Here's how the part is built. I have some questions about the finished solid (model axes, mm). A direction names the side the tool comes from. Round coordinates to 2 decimals unless told otherwise and drop trailing zeros. Order: outer loops, then holes, each group sorted by start corner. A loop starts at its lowest first (then second) coordinate and runs counter-clockwise, first axis right, second up. Notation, with made-up numbers: (-20.75, 15) -> (38.25, 15) arc R10 ccw to (38.25, 19) -> close; hole circle Ø9 at (68, 79). An arc over 180 degrees is marked (long way). Answer in a Markdown table with one row per item.
```python
from build123d import *

# Parameters (mm, degrees)
F0_W     = 80
F0_H     = 50
F1_DEPTH = 60
F2_SIZE  = 20
F4_D     = 16
F4_DEPTH = 10
F4_TIP   = 4.8068849522
F5_R     = 2
F6_R     = 2


with BuildPart() as f1:
    # F0 (on Top) → F1 (new body)
    with BuildSketch(Plane.XY):
        with Locations((40, 25)):
            Rectangle(F0_W, F0_H)
    extrude(amount=F1_DEPTH)

    # F2
    f2_edges = [f1.edges().sort_by_distance(p)[0] for p in [
        (40, 0, 60),
    ]]
    chamfer(f2_edges, length=F2_SIZE)

    # F4
    with Locations(Plane(origin=(0, -20, 20), x_dir=(1, 0, 0), z_dir=(0, -0.7071067812, 0.7071067812))):
        with Locations((20, 42.5685424949), (60, 42.5685424949)):
            Hole(F4_D / 2, depth=F4_DEPTH)
            with Locations((0, 0, -(F4_DEPTH + F4_TIP / 2))):  # 118° drill point
                Cone(0, F4_D / 2, F4_TIP, mode=Mode.SUBTRACT)

    # F5
    f5_edges = [f1.edges().sort_by_distance(p)[0] for p in [
        (80, 25, 0),
    ]]
    fillet(f5_edges, radius=F5_R)

    # F6
    f6_edges = [f1.edges().sort_by_distance(p)[0] for p in [
        (0, 25, 0),
    ]]
    fillet(f6_edges, radius=F6_R)


solid = f1.part
```
1. For faces 5 (the face through (20.75, 20.81, 41.05)), 6 (the face through (39, 10, 50)), which set-ups out of +Z, -Z, +X, -X, +Y, -Y let a thin tool reach every point of the face, with its end or its side?
Numbers:
| item | result |
|---|---|
| face 5 | none |
| face 6 | +Z, +X, -X, -Y |
2. Suppose I cut it at A-A on x = 72. Write out the boundary of the cut face in (y, z).
Numbers:
| item | result |
|---|---|
| outline | (0, 0) -> (50, 0) -> (50, 60) -> (20, 60) -> (0, 40) -> close |
3. We'd pull the mould along X, two halves only. Please class faces 1 (the face through (79.4, 25.35, 0.57)), 2 (the face through (39, 50, 30)), 3 (the face through (58.976, 20.644, 40.885)), 4 (the face through (61.734, 8.163, 40.993)): released by +X, released by -X, zero draft, split by the parting line, or undercut.
Numbers:
| item | result |
|---|---|
| face 1 | released by +X |
| face 2 | zero draft |
| face 3 | undercut |
| face 4 | undercut |
4. Please list where these lines run through material, in increasing order: line 1 along Y through (x, z) = (19.5, 53); line 2 along Y through (x, z) = (45, 49); line 3 along Z through (x, y) = (14.5, 10.5).
Numbers:
| item | result |
|---|---|
| line 1 | y = 18.49 to 50 |
| line 2 | y = 9 to 50 |
| line 3 | z = 0 to 41.49 |
5. For pin 1 Ø8 at (x, y) = (61.5, 14.5) entering from +Z, with a flat end and sliding along its axis, tell me the tip position at first contact or that it passes through.
Numbers:
| item | result |
|---|---|
| pin 1 | stops at z = 58.5 |
